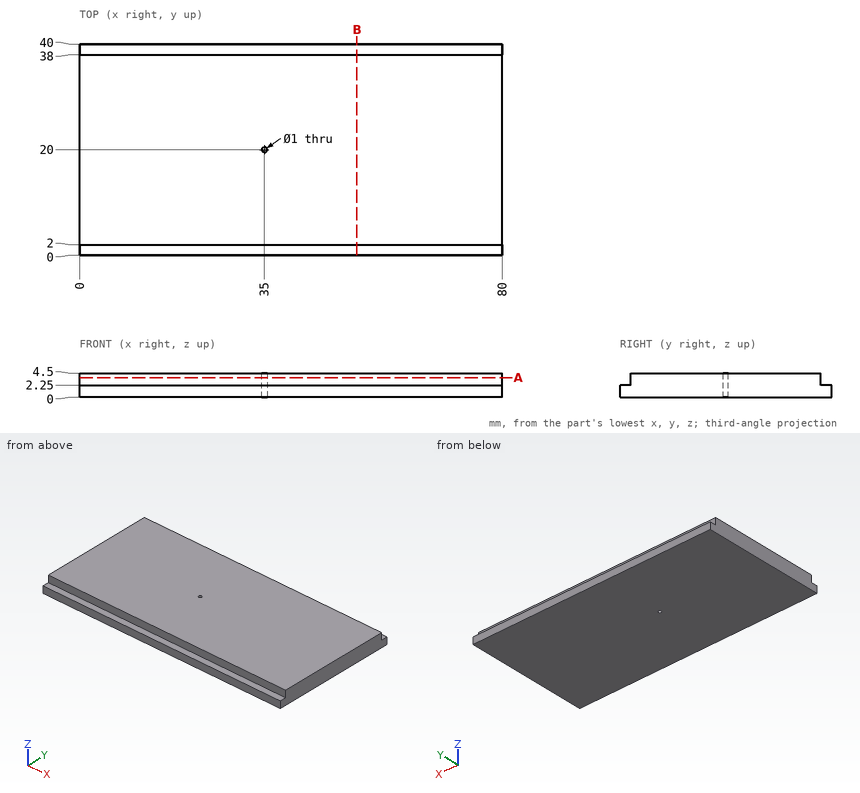
Can you work these out from the drawing? Everything is in mm from the part's minimum corner. Round coordinates to 2 decimals unless told otherwise and drop trailing zeros. Write each loop counter-clockwise with the first axis right and the second up, starting at its lowest first coordinate (ties: lowest second). Pieces come first, ordered by that corner, then holes. Notation, with made-up numbers: M -28.75,-23 L -6.75,-23 A17 ccw -6.75,2 Z; hole C 36,-25 d11. An arc over 180 degrees is marked long. Use a Markdown table: item, result.
Item 1: I want a section at B-B (x = 52.5). List the corners of the cut face in (y, z) for me, and give its area (3 significant figures).
Found:
| item | result |
|---|---|
| outline | M 0,0 L 40,0 L 40,2.25 L 38,2.25 L 38,4.5 L 2,4.5 L 2,2.25 L 0,2.25 Z |
| area | 171 mm2 |
Item 2: I want a section at A-A (z = 3.7). List the corners of the cut face in (x, y) for me, and give its area (3 significant figures).
Found:
| item | result |
|---|---|
| outline | M 0,2 L 80,2 L 80,38 L 0,38 Z; hole C 35,20 d1 |
| area | 2,880 mm2 |
Item 3: If I drill on line 1 along Y through (x, z) = (35, 1.65); line 2 along Y through (x, z) = (35, 2.55); line 3 along Y through (x, z) = (33.5, 3.45), over which ranges is the centre line in solid material (lowest first)? Write a range as [from, to].
Found:
| item | result |
|---|---|
| line 1 | y = [0, 19.5], [20.5, 40] |
| line 2 | y = [2, 19.5], [20.5, 38] |
| line 3 | y = [2, 38] |
Item 4: For pin 1 Ø1 at (x, z) = (52, 4) entering from +Y; pin 2 Ø2.5 at (x, z) = (44.5, 3) entering from +Y; pin 3 Ø1 at (x, y) = (51, 39) entering from +Z; pin 4 Ø0.7 at (x, z) = (31, 4) entering from -Y, each with a flat end and sliding along its axis, tell me the tip position at first contact or that it passes through.
Found:
| item | result |
|---|---|
| pin 1 | stops at y = 38 |
| pin 2 | stops at y = 40 |
| pin 3 | stops at z = 2.25 |
| pin 4 | stops at y = 2 |
